```python
from build123d import *

# Parameters (mm, degrees)
SKETCH1_W           = 54.7
SKETCH1_H           = 51.4
SKETCH1_W_2         = 51.5
SKETCH1_H_2         = 48.2
SKETCH1_W_3         = 48.3
SKETCH1_H_3         = 45
BOSS_EXTRUDE1_DEPTH = 1.6
SKETCH1_3_W         = 51.5
SKETCH1_3_H         = 48.2
SKETCH1_3_W_2       = 48.3
SKETCH1_3_H_2       = 45
BOSS_EXTRUDE2_DEPTH = 3.2
FILLET1_R           = 2
FILLET2_R           = 0.4


with BuildPart() as part:
    # Sketch1 → Boss-Extrude1 (new body)
    # profile 1 of 3: a face of its own
    with BuildSketch(Plane(origin=(0, 0, 0), x_dir=(1, 0, 0), z_dir=(0, 1, 0))):
        Rectangle(SKETCH1_W, SKETCH1_H)
        Rectangle(SKETCH1_W_2, SKETCH1_H_2, mode=Mode.SUBTRACT)
    # profile 2 of 3: a face of its own
    with BuildSketch(Plane(origin=(0, 0, 0), x_dir=(1, 0, 0), z_dir=(0, 1, 0))):
        Rectangle(SKETCH1_W_2, SKETCH1_H_2)
        Rectangle(SKETCH1_W_3, SKETCH1_H_3, mode=Mode.SUBTRACT)
    # profile 3 of 3: a face of its own
    with BuildSketch(Plane(origin=(0, 0, 0), x_dir=(1, 0, 0), z_dir=(0, 1, 0))):
        Rectangle(SKETCH1_W_3, SKETCH1_H_3)
    extrude(amount=BOSS_EXTRUDE1_DEPTH)

    # Sketch1_3 → Boss-Extrude2 (add)
    with BuildSketch(Plane(origin=(0, 0, 0), x_dir=(1, 0, 0), z_dir=(0, 1, 0))):
        Rectangle(SKETCH1_3_W, SKETCH1_3_H)
        Rectangle(SKETCH1_3_W_2, SKETCH1_3_H_2, mode=Mode.SUBTRACT)
    extrude(amount=BOSS_EXTRUDE2_DEPTH)

    # Fillet1
    fillet1_edges = [part.edges().sort_by_distance(p)[0] for p in [
        (-27.35, 0.8, 25.7),
        (-27.35, 0.8, -25.7),
        (27.35, 0.8, -25.7),
        (27.35, 0.8, 25.7),
    ]]
    fillet(fillet1_edges, radius=FILLET1_R)

    # Fillet2
    fillet2_edges = [part.edges().sort_by_distance(p)[0] for p in [
        (-25.75, 2.4, -24.1),
        (-25.75, 2.4, 24.1),
        (25.75, 2.4, 24.1),
        (25.75, 2.4, -24.1),
    ]]
    fillet(fillet2_edges, radius=FILLET2_R)


solid = part.part
```
Verification items for the finished model (mm, model axes). A direction names the side the tool comes from. Round coordinates to 2 decimals unless told otherwise and drop trailing zeros. Order: outer loops, then holes, each group sorted by start corner. A loop starts at its lowest first (then second) coordinate and runs counter-clockwise, first axis right, second up. Notation, with made-up numbers: (84.5, -13.75) -> (121.5, -13.75) arc R25 ccw to (121.5, -1.75) -> close; hole circle Ø9 at (26, 45.25). An arc over 180 degrees is marked (long way). Put each result on its own line as item: value. Start each with the question number.
(1) Section check B-B (x = 23.5). Enter the section's corners in (y, z).
(2) Depth check by flat-ended pin: pin 1 Ø1.3 at (x, y) = (-8.5, 2.5) entering from +Z; pin 2 Ø1.5 at (x, z) = (-0.5, 16.5) entering from +Y; pin 3 Ø0.5 at (x, y) = (-5, 2.5) entering from -Z. Enter the tip coordinate at first touch or a pass-through.
(3) Material ranges on line 1 along Z through (x, y) = (12.5, 2.45); line 2 along X through (y, z) = (2.2, -15); line 3 along Y through (x, z) = (-18, -3.5), recorded low to high.
(4) Draft check along X on faces 4 (the face through (-26.78, 0.81, -25.1)), 5 (the face through (0, 1.6, 0)), 6 (the face through (0, 0, 0)). Enter one of: +X half, -X half, draft (parallel to the pull), parting line (faces both ways), or undercut.
(5) Tool access check on faces 1 (the face through (0, 2, -24.1)), 2 (the face through (0, 2, 22.5)), 3 (the face through (25.75, 2, 0)). Record the directions out of +Z, -Z, +X, -X, +Y, -Y that give a thin tool (end or side, any length) a straight path to the whole face; none if there is none.
(6) Section check A-A (z = 6.5). Enter the section's corners in (x, y).
Completed:
1. outline: (0, -25.7) -> (1.6, -25.7) -> (1.6, -24.1) -> (3.2, -24.1) -> (3.2, -22.5) -> (1.6, -22.5) -> (1.6, 22.5) -> (3.2, 22.5) -> (3.2, 24.1) -> (1.6, 24.1) -> (1.6, 25.7) -> (0, 25.7) -> close
2. pin 1: stops at z = 24.1
2. pin 2: stops at y = 1.6
2. pin 3: stops at z = -24.1
3. line 1: z = -24.1 to -22.5, 22.5 to 24.1
3. line 2: x = -25.75 to -24.15, 24.15 to 25.75
3. line 3: y = 0 to 1.6
4. face 4: -X half
4. face 5: undercut
4. face 6: draft
5. face 1: -Z, +X, -X, +Y
5. face 2: +Y
5. face 3: +Z, -Z, +X, +Y
6. outline: (-27.35, 0) -> (27.35, 0) -> (27.35, 1.6) -> (25.75, 1.6) -> (25.75, 3.2) -> (24.15, 3.2) -> (24.15, 1.6) -> (-24.15, 1.6) -> (-24.15, 3.2) -> (-25.75, 3.2) -> (-25.75, 1.6) -> (-27.35, 1.6) -> close
